Work out the finished part from the listing and answer in its coordinate system (mm). A direction names the side the tool comes from. Round coordinates to 2 decimals unless told otherwise and drop trailing zeros. Order: outer loops, then holes, each group sorted by start corner. A loop starts at its lowest first (then second) coordinate and runs counter-clockwise, first axis right, second up. Notation, with made-up numbers: (57.5, 52.5) - (77.5, 52.5) arc R30 cw to (77.5, 80.5) - close; hole circle Ø1 at (52, 32). An arc over 180 degrees is marked (long way). Use one line per item in the form item = value. Start each with the question number.
Q1. The part is cut by section D-D on z = 13.75. State how many separate pieces and enclosed holes the cut face has, plus the area to 3 significant figures.
Q2. The part is cut by section A-A on z = 9.5. Determine the outline of the cut face in (x, y), plus the area to 3 significant figures.
Q3. Which of the six approach directions +Z, -Z, +X, -X, +Y, -Y give full straight-line access (tool end or side, diameter ignored) to faces 1 (the flat face through (0, 3, 19)), 2 (the cylindrical face through (-9.93, 3.233, 10.002))?
Q4. The part is cut by section B-B on x = 1. Determine the outline of the cut face in (y, z), plus the area to 3 significant figures.
Q5. Find the intervals of material crossed by line 1 (X direction, y = 6.5, z = 11.5); line 2 (Y direction, x = 1, z = 6); line 3 (X direction, y = 7.5, z = 7.5), in increasing order. Write a range as [from, to].
Q6. Given P1, Ø3, axis at y = 3.343, z = 12.5, coming from the -X side, flat-ended and moving along its own axis, determine where the tip first touches the part or whether it passes through.
Q7. For a pull along X with two mould halves and no side action, classify faces 3 (the cylindrical face through (1.613, 4.694, 9.367)), 4 (the cylindrical face through (-10.05, 4.57, 16.81)), 5 (the flat face through (15, 3, 9)), 6 (the flat face through (0, 10.172, 9)) as +X half, -X half, draft (parallel to the pull), parting line (faces both ways), or undercut.
Q8. The part is cut by section C-C on x = -7.5. Determine the outline of the cut face in (y, z), plus the area to 3 significant figures.
Autodesk Inventor part; units mm, degrees
ref_plane "YZ Plane" through (0, 0, 0) normal (1, 0, 0) x (0, 1, 0)
ref_plane "XZ Plane" through (0, 0, 0) normal (0, 1, 0) x (-1, 0, 0)
ref_plane "XY Plane" through (0, 0, 0) normal (0, 0, 1) x (1, 0, 0)
sketch "Sketch1" plane through (0, 0, 0) normal (0, 0, 1) x (1, 0, 0)
  line L0 (-15, 10.1715) -> (15, 10.1715)
  line L1 (15, 10.1715) -> (15, -10.1715)
  line L2 (15, -10.1715) -> (-15, -10.1715)
  line L3 (-15, -10.1715) -> (-15, 10.1715)
  line L4 (0, 0) -> (0, 4.8999) construction
  line L5 (0, 0) -> (4.2328, 0) construction
  dimension "d2" = 20.343
  dimension "d3" = 30
extrude "Extrusion1" add sketch "Sketch1" along normal blind 19
sketch "Sketch2" plane through (15, -10.1715, 0) normal (1, 0, 0) x (0, 0, -1)
  line L0 (0, 0) -> (-19, 0)
  line L1 (0, 0) -> (-30, 0)
  line L2 (-30, 0) -> (-30, 6.343)
  line L3 (-30, 6.343) -> (0, 6.343)
  line L4 (0, 6.343) -> (0, 0)
  point P0 (0, 10.1715)
  dimension "d4" = 30
  dimension "d5" = 6.343
extrude "Extrusion2" cut sketch "Sketch2" against normal up to next
sketch "Sketch3" plane through (0, 0, 19) normal (0, 0, 1) x (1, 0, 0)
  line L0 (15, 10.1715) -> (-15, 10.1715)
  line L1 (-15, 10.1715) -> (-15, -10.1715)
  line L2 (15, -10.1715) -> (15, 10.1715)
  point P0 (0, 0)
  point P1 (1, 6.1715)
  point P2 (11, 6.1715)
  dimension "d8" = 4
  dimension "d9" = 4
  dimension "d17" = 16
  dimension "d18" = 4
hole "Hole1" at (1, 6.1715, 19) at (11, 6.1715, 19) direction (0, 0, -1) diameter 3.2 end through all
sketch "Sketch4" plane through (-15, -10.1715, 19) normal (-1, 0, 0) x (0, 0, 1)
  circle A0 centre (-6.5, 13.5145) radius 2.5
  point P0 (-19, 10.1715)
hole "Hole2" at (-15, 3.343, 12.5) direction (1, 0, 0) diameter 5 depth 10 tip angle 118
sketch "Sketch6" plane through (0, 0, 19) normal (0, 0, 1) x (1, 0, 0)
  line L0 (-15, 0.843) -> (-15, 5.843)
  point P0 (0, 0)
  point P1 (-10, 3.343)
  point P2 (-15, 3.343)
  dimension "d26" = 5
hole "Hole3" at (-10, 3.343, 19) direction (0, 0, -1) diameter 2.459 depth 6.05 tip angle 118
properties part number "3d_LM-Welding_Tooling -  Moving Block" material "Aluminium 6061-T6"
Found:
q1.separate_pieces = 1
q1.enclosed_holes = 2
q1.area = 359 mm²
q2.outline = (-15, -3.83) - (15, -3.83) - (15, 10.17) - (-15, 10.17) - close; hole circle Ø3.2 at (1, 6.17); hole circle Ø3.2 at (11, 6.17)
q2.area = 404 mm²
q3.face_1 = +Z, +X, -X, +Y, -Y
q3.face_2 = -X
q4.outline = (-3.83, 0) - (4.57, 0) - (4.57, 19) - (-3.83, 19) - close; (7.77, 0) - (10.17, 0) - (10.17, 19) - (7.77, 19) - close
q4.area = 205 mm²
q5.line_1 = [-15, -0.57], [2.57, 9.43], [12.57, 15]
q5.line_2 = [-3.83, 4.57], [7.77, 10.17]
q5.line_3 = [-15, 0.11], [1.89, 10.11], [11.89, 15]
q6.P1 = -4.4
q7.face_3 = undercut
q7.face_4 = undercut
q7.face_5 = +X half
q7.face_6 = draft
q8.outline = (-3.83, 0) - (10.17, 0) - (10.17, 19) - (-3.83, 19) - close; hole circle Ø5 at (3.34, 12.5)
q8.area = 246 mm²
